The drawing under review shows one solid part. Ordinate dimensions are in mm from its lowest x, y, z. Round coordinates to 2 decimals unless told otherwise and drop trailing zeros. Write each loop counter-clockwise with the first axis right and the second up, starting at its lowest first coordinate (ties: lowest second). Pieces come first, ordered by that corner, then holes.
Item 1: Add section C-C (z = 140). Give the boundary of the cut face in (x, y), plus the area to 3 significant figures.
Item 2: Add section A-A (x = 30). Give the boundary of the cut face in (y, z), plus the area to 3 significant figures.
Item 3: To check wall thickness, follow L1, parallel to Z at x = 14.5, y = 5.25; L2, parallel to X at y = 5.25, z = 146; L3, parallel to X at y = 7.75, z = 265. State the ranges of each line that lie inside material, in increasing order.
Item 4: Add section B-B (y = 5). Give the boundary of the cut face in (x, z).
Item 5: Clearance check with flat-ended pins moving along their axes: pin 1 Ø3 at (y, z) = (3.5, 141.5) entering from +X; pin 2 Ø3 at (y, z) = (4, 10) entering from +X; pin 3 Ø3 at (y, z) = (2.5, 145) entering from -X. State where each tip first meets the part, or that it passes through.
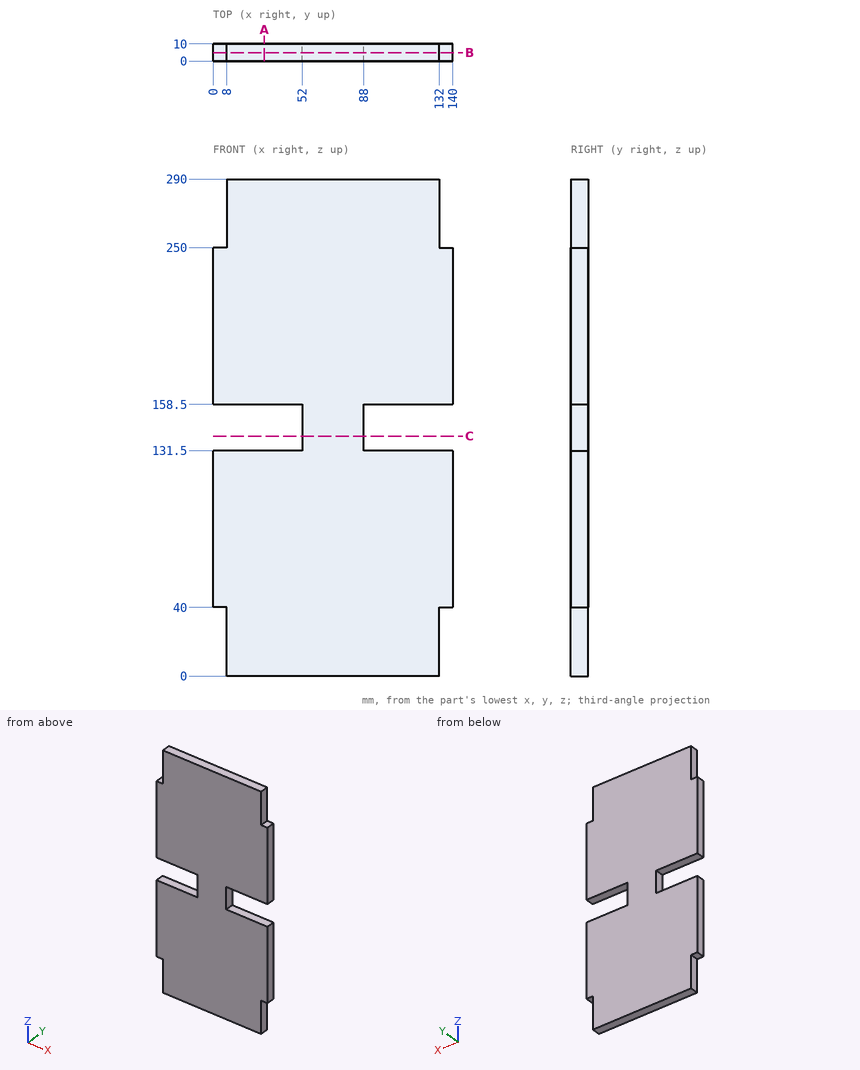
Numbers:
1. outline: (52, 0) - (88, 0) - (88, 10) - (52, 10) - close
1. area: 360 mm2
2. outline: (0, 0) - (10, 0) - (10, 131.5) - (0, 131.5) - close; (0, 158.5) - (10, 158.5) - (10, 290) - (0, 290) - close
2. area: 2,630 mm2
3. L1: z = 0 to 131.5, 158.5 to 290
3. L2: x = 52 to 88
3. L3: x = 8 to 132
4. outline: (0, 40) - (8, 40) - (8, 0) - (132, 0) - (132, 40) - (140, 40) - (140, 131.5) - (88, 131.5) - (88, 158.5) - (140, 158.5) - (140, 250) - (132, 250) - (132, 290) - (8, 290) - (8, 250) - (0, 250) - (0, 158.5) - (52, 158.5) - (52, 131.5) - (0, 131.5) - close
5. pin 1: stops at x = 88
5. pin 2: stops at x = 132
5. pin 3: stops at x = 52
